from build123d import *

# Parameters (mm, degrees)
SKETCH1_W           = 152.4
SKETCH1_H           = 63.5
SKETCH1_R           = 3.175
BOSS_EXTRUDE1_DEPTH = 12.7
SKETCH2_W           = 12.7
SKETCH2_H           = 25.4
CUT_EXTRUDE1_DEPTH  = 153.4


with BuildPart() as part:
    # Sketch1 → Boss-Extrude1 (new body)
    with BuildSketch(Plane.XY):
        Rectangle(SKETCH1_W, SKETCH1_H)
        with Locations((-63.5, 19.05)):
            Circle(SKETCH1_R, mode=Mode.SUBTRACT)
        with Locations((63.5, 19.05)):
            Circle(SKETCH1_R, mode=Mode.SUBTRACT)
        with Locations((63.5, -19.05)):
            Circle(SKETCH1_R, mode=Mode.SUBTRACT)
        with Locations((-63.5, -19.05)):
            Circle(SKETCH1_R, mode=Mode.SUBTRACT)
        with BuildLine():
            Line((-50.8, 6.35), (50.8, 6.35))
            ThreePointArc((50.8, 6.35), (57.15, 0), (50.8, -6.35))
            Line((50.8, -6.35), (-50.8, -6.35))
            ThreePointArc((-50.8, -6.35), (-57.15, 0), (-50.8, 6.35))
        make_face(mode=Mode.SUBTRACT)
    extrude(amount=BOSS_EXTRUDE1_DEPTH)

    # Sketch2 → Cut-Extrude1 (cut, through all)
    with BuildSketch(Plane.ZY.offset(76.2)):
        Rectangle(SKETCH2_W, SKETCH2_H)
    extrude(amount=-CUT_EXTRUDE1_DEPTH, mode=Mode.SUBTRACT)


solid = part.part
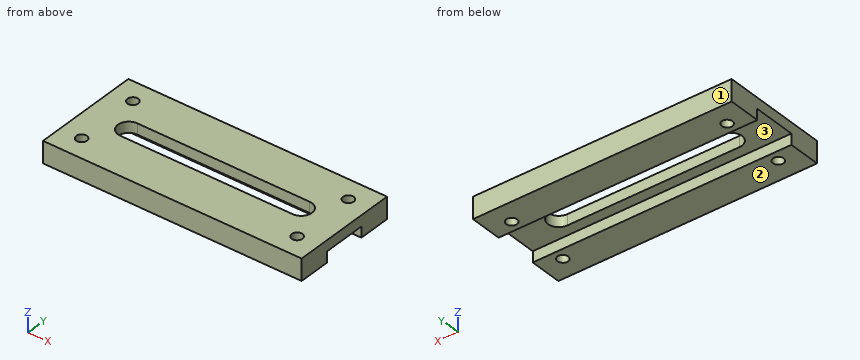
Input: part model. Units: mm. Frame: model coordinates. Face numbers are marked on the shaded views. Coordinates: 2 decimals unless noted, no trailing zeros. Order: outer loops, then holes, each group sorted by start corner. A loop starts at its lowest first (then second) coordinate and runs counter-clockwise, first axis right, second up.
1. Ray query, line 1 along Y through (x, z) = (-63.5, 2.75) (3 decimals); line 2 along Y through (x, z) = (63.5, 8.5) (3 decimals); line 3 along X through (y, z) = (19, 12.25). Return the intervals inside material, ascending.
Checked values:
line 1: y = -31.75 to -22.225, -15.875 to -12.7, 12.7 to 15.875, 22.225 to 31.75
line 2: y = -31.75 to -22.225, -15.875 to 15.875, 22.225 to 31.75
line 3: x = -76.2 to -66.67, -60.33 to 60.33, 66.67 to 76.2
2. Cut plane D-D, the plane y = 0. Return loops of the section in (x, z), plus the area to 3 significant figures.
Checked values:
outline: (-76.2, 6.35) - (-57.15, 6.35) - (-57.15, 12.7) - (-76.2, 12.7) - close; (57.15, 6.35) - (76.2, 6.35) - (76.2, 12.7) - (57.15, 12.7) - close
area: 242 mm2
3. Cut plane A-A, the plane z = 3.5. Return loops of the section in (x, y) (3 decimals), plus the area to 3 significant figures.
Checked values:
outline: (-76.2, -31.75) - (76.2, -31.75) - (76.2, -12.7) - (-76.2, -12.7) - close; (-76.2, 12.7) - (76.2, 12.7) - (76.2, 31.75) - (-76.2, 31.75) - close; hole circle Ø6.35 at (-63.5, -19.05); hole circle Ø6.35 at (-63.5, 19.05); hole circle Ø6.35 at (63.5, -19.05); hole circle Ø6.35 at (63.5, 19.05)
area: 5,680 mm2
4. Cut plane C-C, the plane x = -16. Return loops of the section in (y, z).
Checked values:
outline: (-31.75, 0) - (-12.7, 0) - (-12.7, 6.35) - (-6.35, 6.35) - (-6.35, 12.7) - (-31.75, 12.7) - close; (6.35, 6.35) - (12.7, 6.35) - (12.7, 0) - (31.75, 0) - (31.75, 12.7) - (6.35, 12.7) - close
5. Draft query along Y for the marked faces 1, 2 and 3. Return one class per face: +Y half, -Y half, draft (parallel to the pull), parting line (faces both ways), or undercut.
Checked values:
face 1: +Y half
face 2: draft
face 3: undercut
6. Cut plane B-B, the plane y = -19.05. Return loops of the section in (x, z) (3 decimals), plus the area to 3 significant figures.
Checked values:
outline: (-76.2, 0) - (-66.675, 0) - (-66.675, 12.7) - (-76.2, 12.7) - close; (-60.325, 0) - (60.325, 0) - (60.325, 12.7) - (-60.325, 12.7) - close; (66.675, 0) - (76.2, 0) - (76.2, 12.7) - (66.675, 12.7) - close
area: 1,770 mm2
7. Contact query for flat-ended pins moving along their axis: P1, Ø20.5, axis at x = 37.5, y = -4, coming from the -Z side; P2, Ø1, axis at x = -17, y = -7, coming from the -Z side. Output: stop coordinate, or through.
Checked values:
P1: stops at z = 0
P2: stops at z = 6.35
